```python
from build123d import *

# Parameters (mm, degrees)
SALIENTE_EXTRUIR1_DEPTH = 176


with BuildPart() as part:
    # Croquis1 → Saliente-Extruir1 (new, symmetric)
    with BuildSketch(Plane.XY):
        with BuildLine():
            Line((-9.336754447, -6.045584816), (-12.2, -7))
            Line((-12.2, -7), (-12.2, -0.5))
            ThreePointArc((-12.2, -0.5), (-12.053553391, -0.146446609), (-11.7, 0))
            Line((-11.7, 0), (11.7, 0))
            ThreePointArc((11.7, 0), (12.053553391, -0.146446609), (12.2, -0.5))
            Line((12.2, -0.5), (12.2, -7))
            Line((12.2, -7), (9.336754447, -6.045584816))
            ThreePointArc((9.336754447, -6.045584816), (9.237751563, -5.972790213), (9.2, -5.855848156))
            Line((9.2, -5.855848156), (9.2, -5.277485177))
            ThreePointArc((9.2, -5.277485177), (9.283057943, -5.11523674), (9.463245553, -5.087748518))
            Line((9.463245553, -5.087748518), (11.2, -5.666666667))
            Line((11.2, -5.666666667), (11.2, -1.5))
            ThreePointArc((11.2, -1.5), (11.053553391, -1.146446609), (10.7, -1))
            Line((10.7, -1), (-10.7, -1))
            ThreePointArc((-10.7, -1), (-11.053553391, -1.146446609), (-11.2, -1.5))
            Line((-11.2, -1.5), (-11.2, -5.666666667))
            Line((-11.2, -5.666666667), (-9.463245553, -5.087748518))
            ThreePointArc((-9.463245553, -5.087748518), (-9.283057943, -5.11523674), (-9.2, -5.277485177))
            Line((-9.2, -5.277485177), (-9.2, -5.855848156))
            ThreePointArc((-9.2, -5.855848156), (-9.237751563, -5.972790213), (-9.336754447, -6.045584816))
        make_face()
    extrude(amount=SALIENTE_EXTRUIR1_DEPTH, both=True)


solid = part.part
```
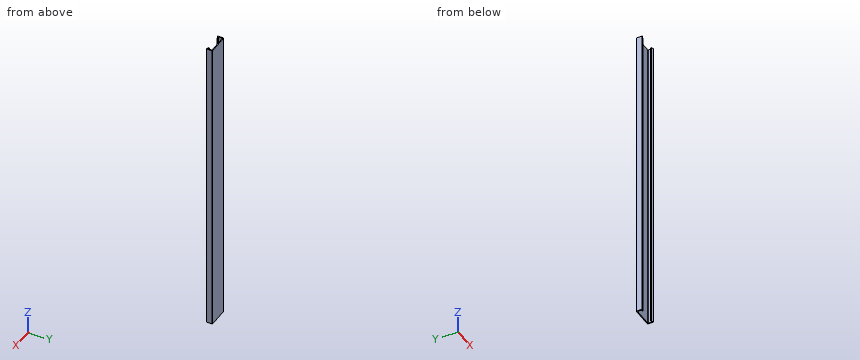
Geometry: final body of the model. Coordinates: model frame, mm. Give positions to 0.01 mm unless a question says otherwise; leave off trailing zeros. Write each loop counter-clockwise with the first axis right and the second up, starting at its lowest first coordinate (ties: lowest second). Pieces come first, ordered by that corner, then holes.
1. Section query A-A, the plane z = 37. Return loops of the section in (x, y).
2. Section query B-B, the plane y = -3.75. Return loops of the section in (x, z), then the cut area to 3 significant figures.
3. Section query C-C, the plane x = -2.75. Return loops of the section in (y, z), then the cut area to 3 significant figures.
4. Pin query (flat end, axial travel): P1, Ø2, axis at x = 6.5, z = -119, coming from the -Y side. Return the tip coordinate at first contact, or that it passes through.
5. Line query: probe 1 along X at (y, z) = (-5.75, 12.5); probe 2 along X at (y, z) = (-2, -161); probe 3 along Y at (x, z) = (6.75, 37). Output: solid intervals per line, ascending.
Computed:
1. outline: (-12.2, -7) - (-9.34, -6.05) arc R0.2 ccw to (-9.2, -5.86) - (-9.2, -5.28) arc R0.2 ccw to (-9.46, -5.09) - (-11.2, -5.67) - (-11.2, -1.5) arc R0.5 cw to (-10.7, -1) - (10.7, -1) arc R0.5 cw to (11.2, -1.5) - (11.2, -5.67) - (9.46, -5.09) arc R0.2 ccw to (9.2, -5.28) - (9.2, -5.86) arc R0.2 ccw to (9.34, -6.05) - (12.2, -7) - (12.2, -0.5) arc R0.5 ccw to (11.7, 0) - (-11.7, 0) arc R0.5 ccw to (-12.2, -0.5) - close
2. outline: (-12.2, -176) - (-11.2, -176) - (-11.2, 176) - (-12.2, 176) - close; (11.2, -176) - (12.2, -176) - (12.2, 176) - (11.2, 176) - close
2. area: 704 mm2
3. outline: (-1, -176) - (0, -176) - (0, 176) - (-1, 176) - close
3. area: 352 mm2
4. P1: stops at y = -1
5. probe 1: x = -12.2 to -9.2, 9.2 to 12.2
5. probe 2: x = -12.2 to -11.2, 11.2 to 12.2
5. probe 3: y = -1 to 0
